```python
from build123d import *

# Parameters (mm, degrees)
F1_DEPTH  = 365
F2_W      = 730
F2_H      = 82.1332173976
F3_DEPTH  = 30
F4_R      = 9
F5_DEPTH  = 604.101
F7_R      = 75
F8_DEPTH  = 15
F10_R     = 75
F11_DEPTH = 15
F13_R     = 75
F14_DEPTH = 15
F15_W     = 800
F15_H     = 1600
F16_DEPTH = 30
F18_DEPTH = 600
F19_R     = 7
F19_R_2   = 9
F20_DEPTH = 31
F21_R     = 9
F22_DEPTH = 31


with BuildPart() as f1:
    # F0 (on Right) → F1 (new body, symmetric)
    with BuildSketch(Plane.YZ):
        with BuildLine():
            ThreePointArc((613.3667826024, -30), (0, -614.1), (-613.3667826024, -30))
            Line((-613.3667826024, -30), (-633.38993519, -30))
            ThreePointArc((-633.38993519, -30), (0, -634.1), (633.38993519, -30))
            Line((633.38993519, -30), (613.3667826024, -30))
        make_face()
    extrude(amount=F1_DEPTH, both=True)

    # F2 (on face) → F3 (join)
    with BuildSketch(Plane.XY.offset(-30)):
        with Locations((0, 654.4333913012)):
            Rectangle(F2_W, F2_H)
        with Locations((0, -654.4333913012)):
            Rectangle(F2_W, F2_H)
    extrude(amount=-F3_DEPTH)

    # F4 (on face) → F5 (cut, through all)
    with BuildSketch(Plane.XY.offset(-30)):
        with Locations((-335, 665.5)):
            Circle(F4_R)
        with Locations((-265, 665.5)):
            Circle(F4_R)
        with Locations((-35, 665.5)):
            Circle(F4_R)
        with Locations((35, 665.5)):
            Circle(F4_R)
        with Locations((265, 665.5)):
            Circle(F4_R)
        with Locations((335, 665.5)):
            Circle(F4_R)
        with Locations((-265, -665.5)):
            Circle(F4_R)
        with Locations((-335, -665.5)):
            Circle(F4_R)
        with Locations((-35, -665.5)):
            Circle(F4_R)
        with Locations((35, -665.5)):
            Circle(F4_R)
        with Locations((265, -665.5)):
            Circle(F4_R)
        with Locations((335, -665.5)):
            Circle(F4_R)
    extrude(amount=-F5_DEPTH, mode=Mode.SUBTRACT)

    # F7 (on offset) → F8 (join)
    with BuildSketch(Plane(origin=(-292, 0, 0), x_dir=(0, -1, 0), z_dir=(-1, 0, 0))):
        with BuildLine():
            Line((-750, -865), (750, -865))
            Line((750, -865), (750, -612))
            Line((750, -612), (692, -60))
            Line((692, -60), (631.2549484955, -60))
            ThreePointArc((631.2549484955, -60), (0, -634.1), (-631.2549484955, -60))
            Line((-631.2549484955, -60), (-692, -60))
            Line((-692, -60), (-750, -612))
            Line((-750, -612), (-750, -865))
        make_face()
        with Locations((-275, -750)):
            Circle(F7_R, mode=Mode.SUBTRACT)
        with Locations((275, -750)):
            Circle(F7_R, mode=Mode.SUBTRACT)
    extrude(amount=F8_DEPTH)

    # F10 (on offset) → F11 (join)
    with BuildSketch(Plane.YZ.offset(8)):
        with BuildLine():
            Line((692, -60), (631.2549484955, -60))
            ThreePointArc((631.2549484955, -60), (0, -634.1), (-631.2549484955, -60))
            Line((-631.2549484955, -60), (-692, -60))
            Line((-692, -60), (-750, -612))
            Line((-750, -612), (-750, -865))
            Line((-750, -865), (750, -865))
            Line((750, -865), (750, -612))
            Line((750, -612), (692, -60))
        make_face()
        with Locations((-275, -750)):
            Circle(F10_R, mode=Mode.SUBTRACT)
        with Locations((275, -750)):
            Circle(F10_R, mode=Mode.SUBTRACT)
    extrude(amount=-F11_DEPTH)

    # F13 (on offset) → F14 (join)
    with BuildSketch(Plane(origin=(293, 0, 0), x_dir=(0, -1, 0), z_dir=(-1, 0, 0))):
        with BuildLine():
            Line((750, -865), (750, -612))
            Line((750, -612), (692, -60))
            Line((692, -60), (631.2549484955, -60))
            ThreePointArc((631.2549484955, -60), (0, -634.1), (-631.2549484955, -60))
            Line((-631.2549484955, -60), (-692, -60))
            Line((-692, -60), (-750, -612))
            Line((-750, -612), (-750, -865))
            Line((-750, -865), (750, -865))
        make_face()
        with Locations((-275, -750)):
            Circle(F13_R, mode=Mode.SUBTRACT)
        with Locations((275, -750)):
            Circle(F13_R, mode=Mode.SUBTRACT)
    extrude(amount=F14_DEPTH)

    # F15 (on face) → F16 (join)
    with BuildSketch(Plane(origin=(0, 0, -865), x_dir=(1, 0, 0), z_dir=(0, 0, -1))):
        Rectangle(F15_W, F15_H)
    extrude(amount=F16_DEPTH)

    # F17 (on face) → F18 (join, through all)
    with BuildSketch(Plane(origin=(-307, 0, 0), x_dir=(0, -1, 0), z_dir=(-1, 0, 0))):
        with BuildLine():
            Line((-434, -462.3059701107), (-596.6989490625, -865))
            Line((-596.6989490625, -865), (-580.5209279224, -865))
            Line((-580.5209279224, -865), (-422.1895378001, -473.1160578253))
            ThreePointArc((-422.1895378001, -473.1160578253), (-428.1288890728, -467.7482916498), (-434, -462.3059701107))
        make_face()
        with BuildLine():
            Line((596.6989490625, -865), (434, -462.3059701107))
            ThreePointArc((434, -462.3059701107), (428.1288890728, -467.7482916498), (422.1895378001, -473.1160578253))
            Line((422.1895378001, -473.1160578253), (580.5209279224, -865))
            Line((580.5209279224, -865), (596.6989490625, -865))
        make_face()
    extrude(amount=-F18_DEPTH)

    # F19 (on face) → F20 (cut)
    with BuildSketch(Plane(origin=(0, 0, -895), x_dir=(1, 0, 0), z_dir=(0, 0, -1))):
        with Locations((-353, 0)):
            Circle(F19_R)
        with Locations((353, 0)):
            Circle(F19_R)
        with Locations((-353, 640)):
            Circle(F19_R)
        with Locations((-240, 753)):
            Circle(F19_R)
        with Locations((-85, 725)):
            Circle(F19_R_2)
        with Locations((85, 725)):
            Circle(F19_R_2)
        with Locations((240, 753)):
            Circle(F19_R)
        with Locations((353, 640)):
            Circle(F19_R)
        with Locations((-353, -640)):
            Circle(F19_R)
        with Locations((-240, -753)):
            Circle(F19_R)
        with Locations((-85, -725)):
            Circle(F19_R_2)
        with Locations((85, -725)):
            Circle(F19_R_2)
        with Locations((353, -640)):
            Circle(F19_R)
        with Locations((240, -753)):
            Circle(F19_R)
    extrude(amount=-F20_DEPTH, mode=Mode.SUBTRACT)

    # F21 (on face) → F22 (cut)
    with BuildSketch(Plane(origin=(0, 0, -895), x_dir=(1, 0, 0), z_dir=(0, 0, -1))):
        with Locations((-125, 685)):
            Circle(F21_R)
        with Locations((-125, 515)):
            Circle(F21_R)
        with Locations((125, 685)):
            Circle(F21_R)
        with Locations((125, 515)):
            Circle(F21_R)
        with Locations((-125, 85)):
            Circle(F21_R)
        with Locations((125, 85)):
            Circle(F21_R)
        with Locations((-125, -85)):
            Circle(F21_R)
        with Locations((125, -85)):
            Circle(F21_R)
        with Locations((-125, -685)):
            Circle(F21_R)
        with Locations((125, -685)):
            Circle(F21_R)
        with Locations((125, -515)):
            Circle(F21_R)
        with Locations((-125, -515)):
            Circle(F21_R)
    extrude(amount=-F22_DEPTH, mode=Mode.SUBTRACT)


solid = f1.part
```
Geometry check sheet. Reference: the model listing, model coordinates, mm. A direction names the side the tool comes from. Round coordinates to 2 decimals unless told otherwise and drop trailing zeros. Use a Markdown table: item, result. Add a question column.
1) Thickness scan on line 1 along X through (y, z) = (-685, -884.75); line 2 along X through (y, z) = (465, -843); line 3 along Y through (x, z) = (-353, -883). Record the ranges inside material, lowest first.
2) Mould release check, pull along Z, two halves, no side actions. Record for faces 4 (the flat face through (-151.5, 514.21, -660.83)), 5 (the flat face through (5, -654, -30)), 6 (the flat face through (-400, 11, -880)): released by +Z, released by -Z, zero draft, split by the parting line, or undercut.
3) Set-up check for faces 1 (the flat face through (293, 10, -636)), 2 (the cylindrical face through (-147.5, -570.75, -276.27)), 3 (the flat face through (141.11, -500.247, -666.315)): record each of +Z, -Z, +X, -X, +Y, -Y from which the full face is reachable in a straight line by a thin tool's end or side.
4) Gauge pin test, flat ends, axial feed: P1, Ø9, axis at x = -176.5, z = -52, coming from the +Y side; P2, Ø2, axis at y = 587.5, z = -248, coming from the +X side; P3, Ø12, axis at x = 54, z = -624.5, coming from the -Y side. Record the tip position at first contact, or that the pin passes through.
Established:
| question | item | result |
|---|---|---|
| 1 | line 1 | -400 to -134, -116 to 116, 134 to 400 |
| 1 | line 2 | -307 to -292, -7 to 8, 278 to 293 |
| 1 | line 3 | -800 to -647, -633 to -7, 7 to 633, 647 to 800 |
| 2 | face 4 | undercut |
| 2 | face 5 | released by +Z |
| 2 | face 6 | zero draft |
| 3 | face 1 | +X |
| 3 | face 2 | -Y |
| 3 | face 3 | none |
| 4 | P1 | y = 695.5 |
| 4 | P2 | x = 293 |
| 4 | P3 | y = -501.95 |
